Part model, mm, in its own coordinate system. A direction names the side the tool comes from. Give positions to 0.01 mm unless a question says otherwise; leave off trailing zeros. Order: outer loops, then holes, each group sorted by start corner. A loop starts at its lowest first (then second) coordinate and runs counter-clockwise, first axis right, second up. Notation, with made-up numbers: M -35.5,83.5 L -27.5,83.5 A31 cw -27.5,115.5 Z; hole C 18,4.5 d11. An arc over 180 degrees is marked long. One line per question, with ' | ' between items.
Autodesk Inventor part; units mm, degrees
ref_plane "YZ Plane" through (0, 0, 0) normal (1, 0, 0) x (0, 1, 0)
ref_plane "XZ Plane" through (0, 0, 0) normal (0, 1, 0) x (-1, 0, 0)
ref_plane "XY Plane" through (0, 0, 0) normal (0, 0, 1) x (1, 0, 0)
sketch "Sketch1" plane through (0, 0, 0) normal (0, 1, 0) x (-1, 0, 0)
  circle A0 centre (0, 0) radius 3.15
  circle A1 centre (0, 0) radius 6
  dimension "d0" = 6.3
  dimension "d2" = 12
extrude "Extrusion1" add sketch "Sketch1" along normal blind 14
sketch "Sketch2" plane through (0, 14, 0) normal (0, 1, 0) x (1, 0, 0)
  circle A0 centre (0, 0) radius 2.6288
  circle A1 centre (0, 0) radius 3.15
  circle A2 centre (0, 0) radius 8.5
  dimension "d5" = 17
extrude "Extrusion2" add sketch "Sketch2" against normal blind 3 contours A2
ref_plane "Work Plane1" through (0, 5.5, 0) normal (0, -1, 0) x (1, 0, 0)
mirror "Mirror1" about plane through (0, 5.5, 0) normal (0, -1, 0) of "Extrusion2"
ref_plane "Work Plane2" through (0, 5.5, 0) normal (0, -1, 0) x (1, 0, 0)
properties part number "Belt tensor2"
1. Probe L1, parallel to Z at x = 0, y = 4.75; L2, parallel to Y at x = -5.5, z = -4.75. List the from-to ranges inside material, lowest first. Write a range as from..to.
Worked out:
L1: z = -6..-3.15, 3.15..6 | L2: y = -3..0, 11..14
2. Mould opens along Z. For faces 3 (the flat face through (4, 14, 0)), 4 (the cylindrical face through (-0.208, 5.381, -3.143)), 5 (the cylindrical face through (4.57, 12.521, -7.167)) say: released by +Z, released by -Z, zero draft, split by the parting line, or undercut.
Worked out:
face 3: zero draft | face 4: undercut | face 5: split by the parting line
3. Slice it at C-C on y = -2. Give the cut face in (x, z), then the cut area to 3 significant figures.
Worked out:
outline: C 0,0 d17; hole C 0,0 d6.3 | area: 196 mm2
4. Slice it at D-D on z = 5.25. Give the cut face in (x, y).
Worked out:
outline: M -6.68,-3 L 6.68,-3 L 6.68,0 L 2.9,0 L 2.9,11 L 6.68,11 L 6.68,14 L -6.68,14 L -6.68,11 L -2.9,11 L -2.9,0 L -6.68,0 Z
5. Tool access for faces 1 (the cylindrical face through (4.57, -1.521, 7.167)), 2 (the flat face through (-2, 0, -6)): list every direction of +Z, -Z, +X, -X, +Y, -Y with a clear straight run to the whole face (end or side of a thin tool).
Worked out:
face 1: +Y, -Y | face 2: none
6. Slice it at A-A on z = 2.25. Give the cut face in (x, y), then the cut area to 3 significant figures.
Worked out:
outline: M -8.2,-3 L -2.2,-3 L -2.2,14 L -8.2,14 L -8.2,11 L -5.56,11 L -5.56,0 L -8.2,0 Z; M 2.2,-3 L 8.2,-3 L 8.2,0 L 5.56,0 L 5.56,11 L 8.2,11 L 8.2,14 L 2.2,14 Z | area: 146 mm2
7. Drop flat-ended pins along their axis: pin 1 (10 mm diameter, centred on y = 6.5, z = -2.5, fed in from -X); pin 2 (3 mm diameter, centred on x = 3, y = 9, fed in from -Z). Give the stop position or say it passes through.
Worked out:
pin 1: stops at x = -8.49 | pin 2: stops at z = -5.81
